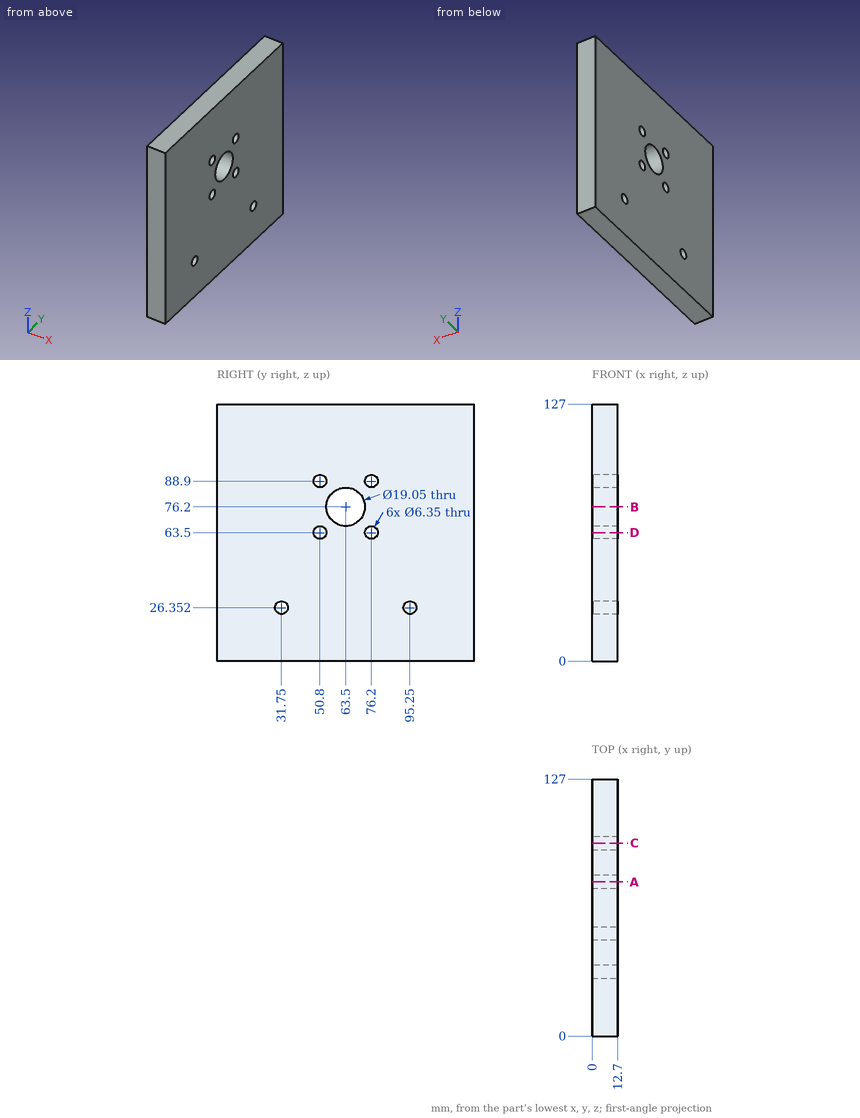
Job drawing, mm, ordinate dimensions from the low corner. One solid piece. Give positions to 0.01 mm unless a question says otherwise; leave off trailing zeros. Write each loop counter-clockwise with the first axis right and the second up, starting at its lowest first coordinate (ties: lowest second). Pieces come first, ordered by that corner, then holes. Notation, with made-up numbers: M 88.5,14.5 L 121.5,14.5 A22 cw 121.5,44.5 Z; hole C 47.25,74 d7. An arc over 180 degrees is marked long. Put each result on its own line as item: value. Start each with the question number.
(1) Band-saw the part on C-C, the plane y = 95.25. Write the cut outline in (x, z).
(2) Band-saw the part on A-A, the plane y = 76.2. Write the cut outline in (x, z) (1 decimal), and give its area (3 significant figures).
(3) Probe L1, parallel to Y at x = 8.5, z = 88.9 (1 decimal); L2, parallel to Z at x = 5.5, y = 76.2 (1 decimal); L3, parallel to Y at x = 6.25, z = 66 (1 decimal). List the from-to ranges inside material, lowest first.
(4) Band-saw the part on B-B, the plane z = 76.2. Write the cut outline in (x, y) (1 decimal), and give its area (3 significant figures).
(5) Band-saw the part on D-D, the plane z = 63.5. Write the cut outline in (x, y) (1 decimal).
Response values:
1. outline: M 0,0 L 12.7,0 L 12.7,23.18 L 0,23.18 Z; M 0,29.53 L 12.7,29.53 L 12.7,127 L 0,127 Z
2. outline: M 0,0 L 12.7,0 L 12.7,60.3 L 0,60.3 Z; M 0,66.7 L 12.7,66.7 L 12.7,85.7 L 0,85.7 Z; M 0,92.1 L 12.7,92.1 L 12.7,127 L 0,127 Z
2. area: 1,450 mm2
3. L1: y = 0 to 47.6, 54 to 73, 79.4 to 127
3. L2: z = 0 to 60.3, 66.7 to 85.7, 92.1 to 127
3. L3: y = 0 to 48.8, 52.8 to 74.2, 78.2 to 127
4. outline: M 0,0 L 12.7,0 L 12.7,54 L 0,54 Z; M 0,73 L 12.7,73 L 12.7,127 L 0,127 Z
4. area: 1,370 mm2
5. outline: M 0,0 L 12.7,0 L 12.7,47.6 L 0,47.6 Z; M 0,54 L 12.7,54 L 12.7,73 L 0,73 Z; M 0,79.4 L 12.7,79.4 L 12.7,127 L 0,127 Z
